Autodesk Fusion 360 part; units mm, degrees
sketch "Sketch1" plane through (0, 0, 0) normal (0, 0, 1) x (1, 0, 0)
  line L0 (0, 30) -> (102.9, 30)
  line L1 (102.9, 30) -> (102.9, -31.8)
  line L2 (102.9, -31.8) -> (0, -31.8)
  line L3 (0, -31.8) -> (0, 30)
  dimension "d1" = 102.9
  dimension "d2" = 61.8
extrude "Extrude1" add sketch "Sketch1" along normal blind 1
sketch "Sketch2" plane through (0, 0, 1) normal (0, 0, 1) x (-1, 0, 0)
  line L0 (0, 31.8) -> (-102.9, 31.8)
  line L1 (-102.9, 31.8) -> (-102.9, -30)
  line L2 (-102.9, -30) -> (0, -30)
  line L3 (0, -30) -> (0, 31.8)
  line L4 (0, 0.9) -> (-102.9, 0.9) construction
  line L5 (-102.9, -28.9) -> (-100.9, -28.9)
  line L6 (-100.9, -28.9) -> (-100.9, 30.7)
  line L7 (-100.9, 30.7) -> (-102.9, 30.7)
  line L8 (-102.9, 30.7) -> (-102.9, -28.9)
  dimension "d6" = 2
  dimension "d9" = 1.1
  dimension "d9" = 1.1
extrude "Extrude2" add sketch "Sketch2" along normal blind 1 contours L1 L5 L6 L7 L8
CAD build for the part. Positions are in the model's coordinates, mm. Give positions to 0.01 mm unless a question says otherwise; leave off trailing zeros. Write each loop counter-clockwise with the first axis right and the second up, starting at its lowest first coordinate (ties: lowest second). Pieces come first, ordered by that corner, then holes. Notation, with made-up numbers: M -16,49.25 L -7,49.25 A35 cw -7,82.25 Z; hole C 20.5,19 d2. An arc over 180 degrees is marked long. Put each result on its own line as item: value. Start each with the question number.
(1) Flat gauge pins, fed straight in: pin 1 Ø8 at (x, y) = (15.5, -6) entering from +Z; pin 2 Ø0.5 at (x, z) = (102.5, 1.5) entering from +Y. Where does each tip first touch, or does it go through?
(2) Band-saw the part on C-C, the plane x = 45. Write the cut outline in (y, z).
(3) Band-saw the part on A-A, the plane y = 12.5. Write the cut outline in (x, z), and give its area (3 significant figures).
(4) Probe L1, parallel to Z at x = 67.5, y = -1.5; L2, parallel to X at y = 6, z = 1.15. List the from-to ranges inside material, lowest first.
(5) Band-saw the part on B-B, the plane z = 1.55. Write the cut outline in (x, y), and give its area (3 significant figures).
Response values:
1. pin 1: stops at z = 1
1. pin 2: stops at y = 28.9
2. outline: M -31.8,0 L 30,0 L 30,1 L -31.8,1 Z
3. outline: M 0,0 L 102.9,0 L 102.9,2 L 100.9,2 L 100.9,1 L 0,1 Z
3. area: 105 mm2
4. L1: z = 0 to 1
4. L2: x = 100.9 to 102.9
5. outline: M 100.9,-30.7 L 102.9,-30.7 L 102.9,28.9 L 100.9,28.9 Z
5. area: 119 mm2
